```python
from build123d import *

# Parameters (mm, degrees)
SKETCH_1_W      = 120
SKETCH_1_H      = 150
SKETCH_1_R      = 1.6
SKETCH_1_R_2    = 1.1
EXTRUDE_1_DEPTH = 4
SKETCH_2_R      = 1.25
EXTRUDE_2_DEPTH = 5
SKETCH_3_R      = 1.2
EXTRUDE_3_DEPTH = 5
FILLET_1_R      = 5
FILLET_3_R      = 3


with BuildPart() as part:
    # 草图1 → 凸台-拉伸1 (new body)
    with BuildSketch(Plane(origin=(0, 0, 0), x_dir=(1, 0, 0), z_dir=(0, 1, 0))):
        Rectangle(SKETCH_1_W, SKETCH_1_H)
        with Locations(Location((-56, 60.1, 0), (0, 0, 270))):
            Circle(SKETCH_1_R, mode=Mode.SUBTRACT)
        with Locations(Location((-56, 14.9, 0), (0, 0, 90))):
            Circle(SKETCH_1_R, mode=Mode.SUBTRACT)
        with Locations(Location((-10, 43.5, 0), (0, 0, 270))):
            Circle(SKETCH_1_R, mode=Mode.SUBTRACT)
        with Locations(Location((-10, 31.5, 0), (0, 0, 90))):
            Circle(SKETCH_1_R, mode=Mode.SUBTRACT)
        with Locations(Location((-56, -14.9, 0), (0, 0, 270))):
            Circle(SKETCH_1_R, mode=Mode.SUBTRACT)
        with Locations(Location((-10, -31.5, 0), (0, 0, 270))):
            Circle(SKETCH_1_R, mode=Mode.SUBTRACT)
        with Locations(Location((-10, -43.5, 0), (0, 0, 90))):
            Circle(SKETCH_1_R, mode=Mode.SUBTRACT)
        with Locations(Location((-56, -60.1, 0), (0, 0, 90))):
            Circle(SKETCH_1_R, mode=Mode.SUBTRACT)
        with Locations(Location((56, -60.1, 0), (0, 0, 270))):
            Circle(SKETCH_1_R, mode=Mode.SUBTRACT)
        with Locations(Location((10, -43.5, 0), (0, 0, 270))):
            Circle(SKETCH_1_R, mode=Mode.SUBTRACT)
        with Locations(Location((10, -31.5, 0), (0, 0, 90))):
            Circle(SKETCH_1_R, mode=Mode.SUBTRACT)
        with Locations(Location((56, -14.9, 0), (0, 0, 90))):
            Circle(SKETCH_1_R, mode=Mode.SUBTRACT)
        with Locations(Location((56, 14.9, 0), (0, 0, 270))):
            Circle(SKETCH_1_R, mode=Mode.SUBTRACT)
        with Locations(Location((10, 31.5, 0), (0, 0, 270))):
            Circle(SKETCH_1_R, mode=Mode.SUBTRACT)
        with Locations(Location((10, 43.5, 0), (0, 0, 90))):
            Circle(SKETCH_1_R, mode=Mode.SUBTRACT)
        with Locations(Location((56, 60.1, 0), (0, 0, 90))):
            Circle(SKETCH_1_R, mode=Mode.SUBTRACT)
        with Locations(Location((0, 8, 0), (0, 0, 270))):
            Circle(SKETCH_1_R_2, mode=Mode.SUBTRACT)
        with Locations(Location((8.8, -8, 0), (0, 0, 270))):
            Circle(SKETCH_1_R_2, mode=Mode.SUBTRACT)
        with Locations(Location((-8.8, -8, 0), (0, 0, 270))):
            Circle(SKETCH_1_R_2, mode=Mode.SUBTRACT)
        with Locations(Location((-25, 8, 0), (0, 0, 270))):
            Circle(SKETCH_1_R, mode=Mode.SUBTRACT)
        with Locations(Location((25, 8, 0), (0, 0, 90))):
            Circle(SKETCH_1_R, mode=Mode.SUBTRACT)
        with Locations(Location((25, -8, 0), (0, 0, 270))):
            Circle(SKETCH_1_R, mode=Mode.SUBTRACT)
        with Locations(Location((-25, -8, 0), (0, 0, 90))):
            Circle(SKETCH_1_R, mode=Mode.SUBTRACT)
        with Locations(Location((35, 70, 0), (0, 0, 270))):
            Circle(SKETCH_1_R, mode=Mode.SUBTRACT)
        with Locations(Location((-35, 70, 0), (0, 0, 90))):
            Circle(SKETCH_1_R, mode=Mode.SUBTRACT)
        with Locations(Location((-35, -70, 0), (0, 0, 270))):
            Circle(SKETCH_1_R, mode=Mode.SUBTRACT)
        with Locations(Location((35, -70, 0), (0, 0, 90))):
            Circle(SKETCH_1_R, mode=Mode.SUBTRACT)
    extrude(amount=EXTRUDE_1_DEPTH)

    # 草图2 → 凸台-拉伸2 (add)
    # profile 1 of 3: a face of its own
    with BuildSketch(Plane.ZY.offset(50)):
        Polygon((45, 0), (75, 0), (75, -7), (57.124355653, -7), align=None)
        with Locations((71, -3.5)):
            Circle(SKETCH_2_R, mode=Mode.SUBTRACT)
        with Locations((65, -3.5)):
            Circle(SKETCH_2_R, mode=Mode.SUBTRACT)
        with Locations((59, -3.5)):
            Circle(SKETCH_2_R, mode=Mode.SUBTRACT)
    # profile 2 of 3: a face of its own
    with BuildSketch(Plane.ZY.offset(50)):
        Polygon((-57.124355653, -7), (-75, -7), (-75, 0), (-45, 0), align=None)
        with Locations((-71, -3.5)):
            Circle(SKETCH_2_R, mode=Mode.SUBTRACT)
        with Locations((-65, -3.5)):
            Circle(SKETCH_2_R, mode=Mode.SUBTRACT)
        with Locations((-59, -3.5)):
            Circle(SKETCH_2_R, mode=Mode.SUBTRACT)
    # profile 3 of 3: a face of its own
    with BuildSketch(Plane.ZY.offset(50)):
        Polygon((-25, 0), (25, 0), (17, -7), (-17, -7), align=None)
    extrude_2 = extrude(amount=-EXTRUDE_2_DEPTH)

    # 镜向1: 凸台-拉伸2 across plane
    add(extrude_2.mirror(Plane.ZY))

    # 草图3 → 凸台-拉伸3 (add)
    with BuildSketch(Plane.XY.offset(75)):
        Polygon((-15, 0), (15, 0), (12, -7), (-12, -7), align=None)
        with Locations((6, -3.5)):
            Circle(SKETCH_3_R, mode=Mode.SUBTRACT)
        with Locations(Location((-6, -3.5, 0), (0, 0, 180))):
            Circle(SKETCH_3_R, mode=Mode.SUBTRACT)
    extrude_3 = extrude(amount=-EXTRUDE_3_DEPTH)

    # 镜向2: 凸台-拉伸3 across plane
    add(extrude_3.mirror(Plane.XY))

    # 圆角1
    fillet_1_edges = [part.edges().sort_by_distance(p)[0] for p in [
        (60, 2, 75),
        (-60, 2, 75),
        (-60, 2, -75),
        (60, 2, -75),
    ]]
    fillet(fillet_1_edges, radius=FILLET_1_R)

    # 圆角3
    fillet_3_edges = [part.edges().sort_by_distance(p)[0] for p in [
        (-47.5, 0, 45),
        (-47.5, -7, 57.124355653),
        (-47.5, -7, 75),
        (47.5, -7, 75),
        (47.5, -7, 57.124355653),
        (47.5, 0, 45),
        (47.5, 0, -45),
        (-47.5, 0, -45),
        (47.5, -7, -75),
        (47.5, -7, -57.124355653),
        (-47.5, -7, -57.124355653),
        (-47.5, -7, -75),
        (-47.5, -7, 17),
        (-47.5, 0, 25),
        (-47.5, 0, -25),
        (-47.5, -7, -17),
        (47.5, 0, -25),
        (47.5, -7, -17),
        (47.5, -7, 17),
        (47.5, 0, 25),
        (-12, -7, -72.5),
        (-15, 0, -72.5),
        (12, -7, -72.5),
        (15, 0, -72.5),
        (-12, -7, 72.5),
        (-15, 0, 72.5),
        (12, -7, 72.5),
        (15, 0, 72.5),
    ]]
    fillet(fillet_3_edges, radius=FILLET_3_R)


solid = part.part
```
Geometry: final body of the model. Coordinates: model frame, mm. A direction names the side the tool comes from. Coordinates: 2 decimals unless noted, no trailing zeros. Order: outer loops, then holes, each group sorted by start corner. A loop starts at its lowest first (then second) coordinate and runs counter-clockwise, first axis right, second up. Notation, with made-up numbers: (31.25, 83) -> (87.25, 83) arc R28 cw to (87.25, 118) -> close; hole circle Ø9 at (75, 61.25). An arc over 180 degrees is marked (long way). Write each question's results on one line, items separated by ' | '. Start each with the question number.
1) Cut plane B-B, the plane z = -3.5. Output: boundary loops of the cut face in (x, y).
2) Cut plane C-C, the plane x = 41. Output: boundary loops of the cut face in (y, z).
3) Set-up query: faces 1 (the cylindrical face through (47.46, -6.1, 74.14)), 2 (the flat face through (50, -3, 0)), 3 (the flat face through (-13.5, -3.5, 72.5)), 4 (the flat face through (47.54, -3.46, -50.99)). Return all of +Z, -Z, +X, -X, +Y, -Y with unobstructed straight access to the full face (end or side cutting, diameter ignored); none if empty.
4) Cut plane A-A, the plane z = 31.5. Output: boundary loops of the cut face in (x, y).
5) Material intervals for line 1 along X through (y, z) = (2.7, 31.5); line 2 along X through (y, z) = (3.25, -8); line 3 along X through (y, z) = (2, -60.1), sorted ascending.
6) First-contact query: pin 1 (10 mm diameter, centred on x = 13.5, z = 39.5, fed in from -Y); pin 2 (5.5 mm diameter, centred on y = -3, z = -55, fed in from +X); pin 3 (6 mm diameter, centred on y = -2, z = -27.5, fed in from -X); pin 4 (2 mm diameter, centred on y = -3.5, z = 71, fed in from -X). Flat tips, straight axial feed; report the tip coordinate or a pass-through.
7) Mould query, pull axis X, two halves, no side actions, for faces 5 (the cylindrical face through (-55.93, 1.97, -61.7)), 6 (the cylindrical face through (58, 2, -74)), 7 (the cylindrical face through (-59, 2, 73)). Classes: released by +X, released by -X, zero draft, split by the parting line, or undercut.
Checks:
1) outline: (-60, 0) -> (-50, 0) -> (-50, -7) -> (-45, -7) -> (-45, 0) -> (45, 0) -> (45, -7) -> (50, -7) -> (50, 0) -> (60, 0) -> (60, 4) -> (-60, 4) -> close
2) outline: (0, -75) -> (4, -75) -> (4, 75) -> (0, 75) -> close
3) face 1: +Z, +X, -Y | face 2: +Z, -Z, +X, -Y | face 3: +Z, -Z, -Y | face 4: +X, -X, -Y
4) outline: (-60, 0) -> (-11.6, 0) -> (-11.6, 4) -> (-60, 4) -> close; (-8.4, 0) -> (8.4, 0) -> (8.4, 4) -> (-8.4, 4) -> close; (11.6, 0) -> (60, 0) -> (60, 4) -> (11.6, 4) -> close
5) line 1: -60 to -11.6, -8.4 to 8.4, 11.6 to 60 | line 2: -60 to -26.6, -23.4 to -1.1, 1.1 to 23.4, 26.6 to 60 | line 3: -60 to -57.6, -54.4 to 54.4, 57.6 to 60
6) pin 1: y = 0 | pin 2: x = 50 | pin 3: x = -60 | pin 4: x = -13.93
7) face 5: undercut | face 6: released by +X | face 7: released by -X
